```python
from build123d import *

# Parameters (mm, degrees)
CROQUIS1_R              = 25
CROQUIS1_R_2            = 1.75
SALIENTE_EXTRUIR1_DEPTH = 8
CROQUIS2_R              = 32.5
CROQUIS2_R_2            = 25
SALIENTE_EXTRUIR2_DEPTH = 10


with BuildPart() as part:
    # Croquis1 → Saliente-Extruir1 (new body)
    with BuildSketch(Plane(origin=(0, 0, 0), x_dir=(1, 0, 0), z_dir=(0, 1, 0))):
        with BuildLine():
            Line((-39.280821918, 2.125330436), (-25.821917808, 19.73521119))
            ThreePointArc((-25.821917808, 19.73521119), (-16.25, 28.145825623), (-4.180235335, 32.230042391))
            Line((-4.180235335, 32.230042391), (17.79982081, 35.08085488))
            ThreePointArc((17.79982081, 35.08085488), (20, 34.641016151), (21.481001108, 32.955524444))
            Line((21.481001108, 32.955524444), (30.002153144, 12.494831201))
            ThreePointArc((30.002153144, 12.494831201), (32.5, 0), (30.002153144, -12.494831201))
            Line((30.002153144, -12.494831201), (21.481001108, -32.955524444))
            ThreePointArc((21.481001108, -32.955524444), (20, -34.641016151), (17.79982081, -35.08085488))
            Line((17.79982081, -35.08085488), (-4.180235335, -32.230042391))
            ThreePointArc((-4.180235335, -32.230042391), (-16.25, -28.145825623), (-25.821917808, -19.73521119))
            Line((-25.821917808, -19.73521119), (-39.280821918, -2.125330436))
            ThreePointArc((-39.280821918, -2.125330436), (-40, 0), (-39.280821918, 2.125330436))
        make_face()
        with Locations(Location((0, 0, 0), (0, 0, 270))):
            Circle(CROQUIS1_R, mode=Mode.SUBTRACT)
        with Locations(Location((18.25, 31.609927238, 0), (0, 0, 270))):
            Circle(CROQUIS1_R_2, mode=Mode.SUBTRACT)
        with Locations(Location((-36.5, 0, 0), (0, 0, 270))):
            Circle(CROQUIS1_R_2, mode=Mode.SUBTRACT)
        with Locations(Location((18.25, -31.609927238, 0), (0, 0, 270))):
            Circle(CROQUIS1_R_2, mode=Mode.SUBTRACT)
    extrude(amount=SALIENTE_EXTRUIR1_DEPTH)

    # Croquis2 → Saliente-Extruir2 (add)
    with BuildSketch(Plane(origin=(0, 8, 0), x_dir=(1, 0, 0), z_dir=(0, 1, 0))):
        with Locations(Location((0, 0, 0), (0, 0, 97.390006376))):
            Circle(CROQUIS2_R)
        with Locations(Location((0, 0, 0), (0, 0, 270))):
            Circle(CROQUIS2_R_2, mode=Mode.SUBTRACT)
    extrude(amount=SALIENTE_EXTRUIR2_DEPTH)


solid = part.part
```
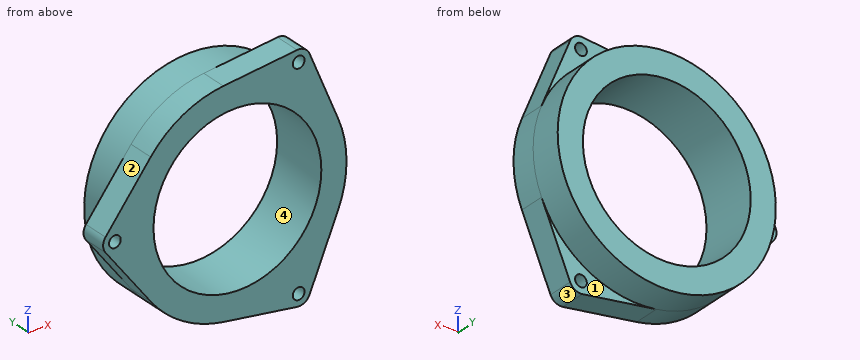
Geometry: final body of the model. Coordinates: model frame, mm. Face numbers are marked on the shaded views. Give positions to 0.01 mm unless a question says otherwise; leave off trailing zeros. Write each loop counter-clockwise with the first axis right and the second up, starting at its lowest first coordinate (ties: lowest second). Pieces come first, ordered by that corner, then holes.
1. Section query B-B, the plane x = 0. Return loops of the section in (y, z).
2. Section query A-A, the plane z = 0. Return loops of the section in (x, y), then the cut area to 3 significant figures.
3. Line query: probe 1 along X at (y, z) = (1, -22); probe 2 along Y at (x, z) = (22, 30); probe 3 along X at (y, z) = (16, 30). Output: solid intervals per line, ascending.
4. Draft query along Z for the marked faces 1, 2, 3 and 4. Return one class per face: released by +Z, released by -Z, zero draft, split by the parting line, or undercut.
5. Pin query (flat end, axial travel): P1, Ø4, axis at x = 18.25, z = 31.61, coming from the +Y side; P2, Ø10, axis at x = -23, y = 15, coming from the -Z side; P3, Ø10, axis at x = -25, z = 8.5, coming from the -Y side; P4, Ø2, axis at x = -24, y = 10, coming from the -Z side. Return the tip coordinate at first contact, or that it passes through.
6. Section query D-D, the plane y = 13. Return loops of the section in (x, z), then the cut area to 3 significant figures.
7. Section query C-C, the plane z = -7.5. Return loops of the section in (x, y).
Computed:
1. outline: (0, -32.77) - (8, -32.77) - (8, -32.5) - (18, -32.5) - (18, -25) - (0, -25) - close; (0, 25) - (18, 25) - (18, 32.5) - (8, 32.5) - (8, 32.77) - (0, 32.77) - close
2. outline: (-40, 0) - (-38.25, 0) - (-38.25, 8) - (-40, 8) - close; (-34.75, 0) - (-25, 0) - (-25, 18) - (-32.5, 18) - (-32.5, 8) - (-34.75, 8) - close; (25, 0) - (32.5, 0) - (32.5, 18) - (25, 18) - close
2. area: 302 mm2
3. probe 1: x = -23.92 to -11.87, 11.87 to 26.04
3. probe 2: y = 0 to 8
3. probe 3: x = -12.5 to 12.5
4. face 1: zero draft
4. face 2: released by +Z
4. face 3: released by -Z
4. face 4: undercut
5. P1: stops at y = 8
5. P2: stops at z = -27.06
5. P3: stops at y = 0
5. P4: stops at z = -22.96
6. outline: circle Ø65 at (0, 0); hole circle Ø50 at (0, 0)
6. area: 1,350 mm2
7. outline: (-35.17, 0) - (-23.85, 0) - (-23.85, 18) - (-31.62, 18) - (-31.62, 8) - (-35.17, 8) - close; (23.85, 0) - (31.62, 0) - (31.62, 18) - (23.85, 18) - close
